Work out the finished part from the listing and answer in its coordinate system (mm). A direction names the side the tool comes from. Coordinates: 2 decimals unless noted, no trailing zeros. Order: outer loops, then holes, each group sorted by start corner. A loop starts at its lowest first (then second) coordinate and runs counter-clockwise, first axis right, second up. Notation, with made-up numbers: M 65,-2.75 L 102,-2.75 A22 ccw 102,13.25 Z; hole C -13.75,42 d1. An arc over 180 degrees is marked long. Answer in a Markdown table with one row per item. Add a question column.
Item 1: A flat-ended cylindrical pin translates along its axis: pin 1 Ø1 at (x, z) = (17, 145) entering from -Y. Find the tip coordinate at first contact, or state that the pin passes through.
Item 2: The part is cut by section A-A (x = 54.5). Write down the section's boundary in (y, z).
Item 3: The mould has two halves that part along Y. Classify faces 1 (the face through (32, 38, 146.05)), 2 (the face through (32, 76.2, 143)), 3 (the face through (55.324, 58.958, 144.446)): released by +Y, released by -Y, zero draft, split by the parting line, or undercut.
Item 4: The part is cut by section D-D (y = 8.5). Write down the section's boundary in (x, z).
Item 5: The part is cut by section B-B (z = 141.75). Write down the section's boundary in (x, y), then the cut area to 3 significant figures.
Item 6: Consider line 1 (X direction, y = 28, z = 143.5); line 2 (X direction, y = 63.5, z = 141.25); line 3 (Z direction, x = 60, y = 50.5). Determine where each line is inside the solid, lowest interval first. Write a range as from..to.
Item 7: Which of the six approach directions +Z, -Z, +X, -X, +Y, -Y give full straight-line access (tool end or side, diameter ignored) to faces 4 (the face through (0, 38, 143)), 5 (the face through (56.557, 42.025, 143.788))?
Item 8: The part is cut by section C-C (y = 20.5). Write down the section's boundary in (x, z), then the cut area to 3 significant figures.
from build123d import *

# Parameters (mm, degrees)
BOSS_EXTRUDE1_DEPTH = 76.2
CUT_EXTRUDE1_DEPTH  = 7.35


with BuildPart() as part:
    # Sketch1 → Boss-Extrude1 (new body)
    with BuildSketch(Plane(origin=(0, 0, 0), x_dir=(1, 0, 0), z_dir=(0, 1, 0))):
        Polygon((0, -146.05), (64.407023089, -146.05), (50.789404144, -139.7), (0, -139.7), align=None)
    extrude(amount=BOSS_EXTRUDE1_DEPTH)

    # Sketch2 → Cut-Extrude1 (cut, through all)
    with BuildSketch(Plane.XY.offset(146.05)):
        Polygon((64.407023089, 0), (64.407023089, 12.7), (51.707023089, 6.35), align=None)
        Polygon((64.407023089, 12.7), (64.407023089, 25.4), (51.707023089, 19.05), align=None)
        Polygon((64.407023089, 25.4), (64.407023089, 38.1), (51.707023089, 31.75), align=None)
        Polygon((64.407023089, 38.1), (64.407023089, 50.8), (51.707023089, 44.45), align=None)
        Polygon((64.407023089, 50.8), (64.407023089, 63.5), (51.707023089, 57.15), align=None)
        Polygon((64.407023089, 63.5), (64.407023089, 76.2), (51.707023089, 69.85), align=None)
    extrude(amount=-CUT_EXTRUDE1_DEPTH, mode=Mode.SUBTRACT)


solid = part.part
Reply:
| question | item | result |
|---|---|---|
| 1 | pin 1 | stops at y = 0 |
| 2 | outline | M 0,141.43 L 4.95,141.43 L 4.95,146.05 L 0,146.05 Z; M 7.75,141.43 L 17.65,141.43 L 17.65,146.05 L 7.75,146.05 Z; M 20.45,141.43 L 30.35,141.43 L 30.35,146.05 L 20.45,146.05 Z; M 33.15,141.43 L 43.05,141.43 L 43.05,146.05 L 33.15,146.05 Z; M 45.85,141.43 L 55.75,141.43 L 55.75,146.05 L 45.85,146.05 Z; M 58.55,141.43 L 68.45,141.43 L 68.45,146.05 L 58.55,146.05 Z; M 71.25,141.43 L 76.2,141.43 L 76.2,146.05 L 71.25,146.05 Z |
| 3 | face 1 | zero draft |
| 3 | face 2 | released by +Y |
| 3 | face 3 | undercut |
| 4 | outline | M 0,139.7 L 50.79,139.7 L 56.01,142.13 L 56.01,146.05 L 0,146.05 Z |
| 5 | outline | M 0,0 L 55.19,0 L 55.19,4.61 L 51.71,6.35 L 55.19,8.09 L 55.19,17.31 L 51.71,19.05 L 55.19,20.79 L 55.19,30.01 L 51.71,31.75 L 55.19,33.49 L 55.19,42.71 L 51.71,44.45 L 55.19,46.19 L 55.19,55.41 L 51.71,57.15 L 55.19,58.89 L 55.19,68.11 L 51.71,69.85 L 55.19,71.59 L 55.19,76.2 L 0,76.2 Z |
| 5 | area | 4,170 mm2 |
| 6 | line 1 | x = 0..58.94 |
| 6 | line 2 | x = 0..54.11 |
| 6 | line 3 | z = 143.99..146.05 |
| 7 | face 4 | +Z, -Z, -X, +Y, -Y |
| 7 | face 5 | +Z, -Z, +X |
| 8 | outline | M 0,139.7 L 50.79,139.7 L 54.61,141.48 L 54.61,146.05 L 0,146.05 Z |
| 8 | area | 343 mm2 |
